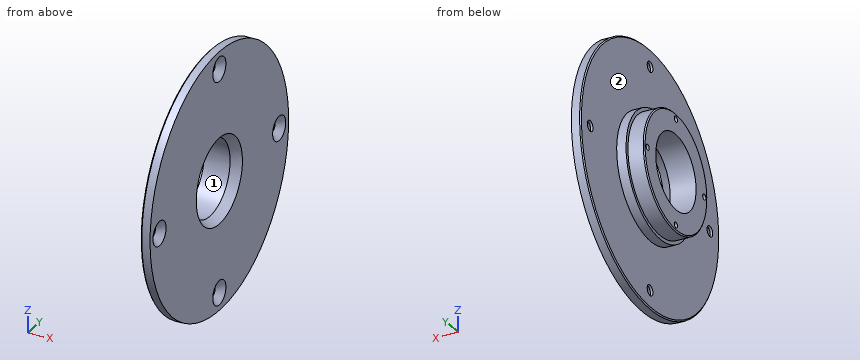
from build123d import *

# Parameters (mm, degrees)
FRAISAGE_POUR_VIS_T_TE_FRAIS_E_M42_D           = 4.5
FRAISAGE_POUR_VIS_T_TE_FRAIS_E_M42_CSINK_D     = 10.4
FRAISAGE_POUR_VIS_T_TE_FRAIS_E_M42_CSINK_ANGLE = 90
CHANFREIN1_SIZE                                = 0.5
TROU_TARAUD_M32_D                              = 2.5
TROU_TARAUD_M32_DEPTH                          = 10.5
TROU_TARAUD_M32_TIP                            = 0.751075774
CHANFREIN2_SIZE                                = 4
CHANFREIN2_SIZE2                               = 2.309401077


with BuildPart() as part:
    # Esquisse1 → Révolution1 (revolve)
    with BuildSketch(Plane.XY, mode=Mode.PRIVATE) as r_volution1_sk:
        Polygon((0, 16), (0, 25), (7, 25), (7, 26.5), (11, 26.5), (11, 55), (15, 55), (15, 16), align=None)
    revolve(r_volution1_sk.sketch.rotate(Axis((0, 0, 0), (1, 0, 0)), 90), axis=Axis((0, 0, 0), (1, 0, 0)))

    # Fraisage pour vis à tête fraisée M42 (through all)
    with Locations(Plane(origin=(15, 0, 0), x_dir=(0, 0, -1), z_dir=(1, 0, 0))):
        with Locations((0, 47.5), (47.5, 0), (0, -47.5), (-47.5, 0)):
            CounterSinkHole(FRAISAGE_POUR_VIS_T_TE_FRAIS_E_M42_D / 2, FRAISAGE_POUR_VIS_T_TE_FRAIS_E_M42_CSINK_D / 2, counter_sink_angle=FRAISAGE_POUR_VIS_T_TE_FRAIS_E_M42_CSINK_ANGLE)

    # Chanfrein1
    chanfrein1_edges = [part.edges().sort_by_distance(p)[0] for p in [
        (11, 0, -55),
        (0, 0, -25),
    ]]
    chamfer(chanfrein1_edges, length=CHANFREIN1_SIZE)

    # Trou taraudé M32
    with Locations(Plane.ZY):
        with Locations((0, 22.5), (-22.5, 0), (0, -22.5), (22.5, 0)):
            Hole(TROU_TARAUD_M32_D / 2, depth=TROU_TARAUD_M32_DEPTH)
            with Locations((0, 0, -(TROU_TARAUD_M32_DEPTH + TROU_TARAUD_M32_TIP / 2))):  # 118° drill point
                Cone(0, TROU_TARAUD_M32_D / 2, TROU_TARAUD_M32_TIP, mode=Mode.SUBTRACT)

    # Chanfrein2
    chanfrein2_edges = [part.edges().sort_by_distance(p)[0] for p in [
        (15, 0, -16),
    ]]
    chanfrein2_side = [part.faces().sort_by_distance(p)[0] for p in [
        (7.5, 0, -16),
    ]]
    chamfer(chanfrein2_edges, length=CHANFREIN2_SIZE, length2=CHANFREIN2_SIZE2, reference=chanfrein2_side[0])


solid = part.part
The listing builds one solid part. Answer for the finished solid, in the listing's coordinates (mm). Face numbers are marked on the shaded views. Give positions to 0.01 mm unless a question says otherwise; leave off trailing zeros. Order: outer loops, then holes, each group sorted by start corner. A loop starts at its lowest first (then second) coordinate and runs counter-clockwise, first axis right, second up. Notation, with made-up numbers: (37, -10) - (58, -10) arc R15 ccw to (58, 1) - close; hole circle Ø11 at (-20, 61). An arc over 180 degrees is marked (long way). One line per item, written item: value. Start each with the question number.
1) Given pin 1 Ø3 at (y, z) = (-3, -16) entering from -X; pin 2 Ø1.5 at (x, z) = (8, -8.5) entering from -Y; pin 3 Ø6 at (x, y) = (12, 31.5) entering from +Z; pin 4 Ø1 at (y, z) = (-14.5, -28) entering from -X, each flat-ended and moving along its own axis, determine where each tip first touches the part or whether it passes through.
2) Find the intervals of material crossed by L1, parallel to Y at x = 5.75, z = 0; L2, parallel to X at y = -36.5, z = -21; L3, parallel to Z at x = 7.5, y = 22.5, in increasing order.
3) The mould has two halves that part along Z. Classify the marked faces 1 and 2: released by +Z, released by -Z, zero draft, split by the parting line, or undercut.
4) A cutting plane is placed at A-A on x = 5. Give the vertices of the cut face in (y, z).
Answer sheet:
1. pin 1: stops at x = 0
1. pin 2: stops at y = -25.34
1. pin 3: stops at z = 47.04
1. pin 4: stops at x = 11
2. L1: y = -25 to -23.75, -21.25 to -16, 16 to 21.25, 23.75 to 25
2. L2: x = 11 to 15
2. L3: z = -14 to -1.25, 1.25 to 14
3. face 1: undercut
3. face 2: zero draft
4. outline: circle Ø50 at (0, 0); hole circle Ø2.5 at (-22.5, 0); hole circle Ø32 at (0, 0); hole circle Ø2.5 at (0, -22.5); hole circle Ø2.5 at (0, 22.5); hole circle Ø2.5 at (22.5, 0)
